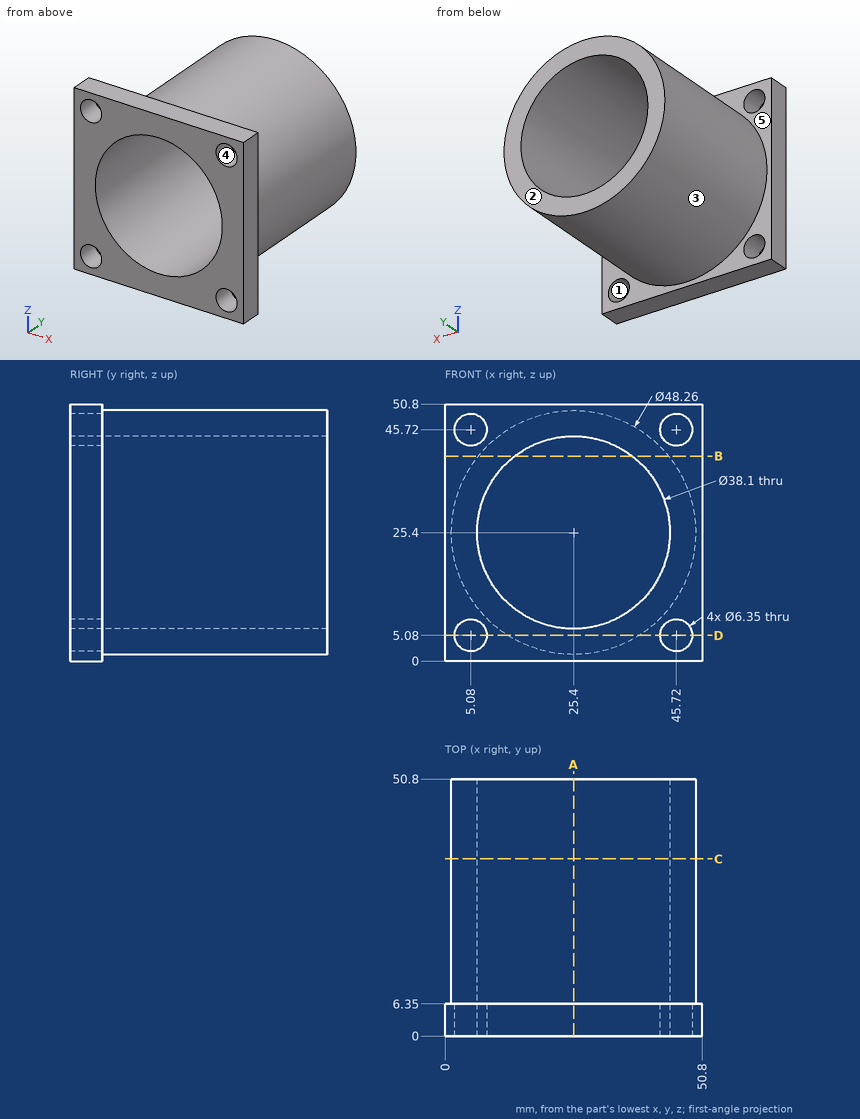
Can you work these out from the drawing? Everything is in mm from the part's minimum corner. A direction names the side the tool comes from. Round coordinates to 2 decimals unless told otherwise and drop trailing zeros. Loops run counter-clockwise (first coordinate to the right, second up) from the corner with the lowest first, then second, coordinate; pieces in that order, holes last. Notation, with made-up numbers: (28.5, -38) - (86.5, -38) arc R30 ccw to (86.5, 1) - close; hole circle Ø7 at (77.25, -35). An arc over 180 degrees is marked (long way). Answer in a Markdown table with one row per item. Add a question column.
(1) If we section it at A-A (x = 25.4): Please give me the cut outline in (y, z).
(2) For the marked faces 4 and 5, which set-ups out of +Z, -Z, +X, -X, +Y, -Y let a thin tool reach every point of the face, with its end or its side?
(3) I'm going to push flat-ended pins straight in: pin 1 (5.5 mm diameter, centred on x = 5.08, z = 45.72, fed in from -Y); pin 2 (6 mm diameter, centred on x = 29, y = 42, fed in from +Z); pin 3 (1 mm diameter, centred on y = 38.5, z = 16, fed in from +X); pin 4 (1.5 mm diameter, centred on y = 11, z = 7.5, fed in from -X). Where does each tip first touch, or does it pass through?
(4) I need wall thicknesses on line 1 along Z through (x, y) = (5.08, 3.5) (3 decimals); line 2 along X through (y, z) = (37, 25); line 3 along Z through (x, y) = (45, 3). Which ranges of each line are inside material? Lowest first, please.
(5) If we mould it in two halves opening along Z, with no side actions, what happens to the marked faces 1, 2 and 3? For each: pulls with the +Z half, pulls with the -Z half, needs draft (parallel to the pull), parting line crosses it, or undercut.
(6) If we section it at B-B (z = 40.5): Please give me the cut outline in (x, y), plus the area to 3 significant figures.
(7) If we section it at C-C (y = 35): Please give me the cut outline in (x, z), plus the area to 3 significant figures.
(8) If we section it at D-D (z = 5.08): Please give me the cut outline in (x, y) (3 decimals), plus the area to 3 significant figures.
Model answer:
| question | item | result |
|---|---|---|
| 1 | outline | (0, 0) - (6.35, 0) - (6.35, 1.27) - (50.8, 1.27) - (50.8, 6.35) - (0, 6.35) - close; (0, 44.45) - (50.8, 44.45) - (50.8, 49.53) - (6.35, 49.53) - (6.35, 50.8) - (0, 50.8) - close |
| 2 | face 4 | +Y, -Y |
| 2 | face 5 | +Y |
| 3 | pin 1 | passes through |
| 3 | pin 2 | stops at z = 49.52 |
| 3 | pin 3 | stops at x = 47.83 |
| 3 | pin 4 | stops at x = 8.43 |
| 4 | line 1 | z = 0 to 1.905, 8.255 to 42.545, 48.895 to 50.8 |
| 4 | line 2 | x = 1.27 to 6.35, 44.45 to 49.53 |
| 4 | line 3 | z = 0 to 1.99, 8.17 to 42.63, 48.81 to 50.8 |
| 5 | face 1 | undercut |
| 5 | face 2 | needs draft |
| 5 | face 3 | parting line crosses it |
| 6 | outline | (0, 0) - (13.79, 0) - (13.79, 50.8) - (6.58, 50.8) - (6.58, 6.35) - (0, 6.35) - close; (37.01, 0) - (50.8, 0) - (50.8, 6.35) - (44.22, 6.35) - (44.22, 50.8) - (37.01, 50.8) - close |
| 6 | area | 816 mm² |
| 7 | outline | circle Ø48.26 at (25.4, 25.4); hole circle Ø38.1 at (25.4, 25.4) |
| 7 | area | 689 mm² |
| 8 | outline | (0, 0) - (1.905, 0) - (1.905, 6.35) - (0, 6.35) - close; (8.255, 0) - (42.545, 0) - (42.545, 6.35) - (38.414, 6.35) - (38.414, 50.8) - (12.386, 50.8) - (12.386, 6.35) - (8.255, 6.35) - close; (48.895, 0) - (50.8, 0) - (50.8, 6.35) - (48.895, 6.35) - close |
| 8 | area | 1,400 mm² |
